```python
from build123d import *

# Parameters (mm, degrees)
SKETCH1_W               = 177.8
SKETCH1_H               = 317.5
BASE_DEPTH              = 6.35
HOLES_DEPTH             = 183.057944073
HOLES_DEPTH_BACK        = 183.057944073
SKETCH3_R               = 3.302
INNER_CUTOUT_DEPTH      = 183.057944073
INNER_CUTOUT_DEPTH_BACK = 183.057944073
FILLET1_R               = 6.35


with BuildPart() as part:
    # Sketch1 → Base (new body)
    with BuildSketch(Plane(origin=(0, 0, 0), x_dir=(1, 0, 0), z_dir=(0, 1, 0))):
        Rectangle(SKETCH1_W, SKETCH1_H)
    extrude(amount=BASE_DEPTH)

    # Sketch3 → Holes (cut, two sides: drawn at the far end of the back side and taken through both)
    with BuildSketch(Plane.XZ.offset(-HOLES_DEPTH_BACK)):
        with Locations(Location((-76.2, -146.05, 0), (0, 0, 270))):
            Circle(SKETCH3_R)
        with Locations(Location((76.2, -146.05, 0), (0, 0, 270))):
            Circle(SKETCH3_R)
        with Locations(Location((76.2, 133.35, 0), (0, 0, 270))):
            Circle(SKETCH3_R)
        with Locations(Location((-76.2, 133.35, 0), (0, 0, 270))):
            Circle(SKETCH3_R)
    extrude(amount=HOLES_DEPTH + HOLES_DEPTH_BACK, mode=Mode.SUBTRACT)

    # Sketch6 → Inner Cutout (cut, two sides: drawn at the far end of the back side and taken through both)
    with BuildSketch(Plane.XZ.offset(-INNER_CUTOUT_DEPTH_BACK)):
        with BuildLine():
            Line((-76.2, 120.65), (-76.2, -133.35))
            ThreePointArc((-76.2, -133.35), (-67.219743879, -137.069743879), (-63.5, -146.05))
            Line((-63.5, -146.05), (63.5, -146.05))
            ThreePointArc((63.5, -146.05), (67.219743879, -137.069743879), (76.2, -133.35))
            Line((76.2, -133.35), (76.2, 120.65))
            ThreePointArc((76.2, 120.65), (67.219743879, 124.369743879), (63.5, 133.35))
            Line((63.5, 133.35), (-63.5, 133.35))
            ThreePointArc((-63.5, 133.35), (-67.219743879, 124.369743879), (-76.2, 120.65))
        make_face()
    extrude(amount=INNER_CUTOUT_DEPTH + INNER_CUTOUT_DEPTH_BACK, mode=Mode.SUBTRACT)

    # Fillet1
    fillet1_edges = [part.edges().sort_by_distance(p)[0] for p in [
        (-76.2, 3.175, 120.65),
        (-63.5, 3.175, 133.35),
        (63.5, 3.175, 133.35),
        (76.2, 3.175, 120.65),
        (76.2, 3.175, -133.35),
        (63.5, 3.175, -146.05),
        (-63.5, 3.175, -146.05),
        (-76.2, 3.175, -133.35),
        (88.9, 3.175, 158.75),
        (-88.9, 3.175, 158.75),
        (-88.9, 3.175, -158.75),
        (88.9, 3.175, -158.75),
    ]]
    fillet(fillet1_edges, radius=FILLET1_R)


solid = part.part
```
Can you work these out from the model? Positions are in its coordinate system, mm. A direction names the side the tool comes from. Round coordinates to 2 decimals unless told otherwise and drop trailing zeros. Order: outer loops, then holes, each group sorted by start corner. A loop starts at its lowest first (then second) coordinate and runs counter-clockwise, first axis right, second up. Notation, with made-up numbers: (-9, 45) -> (42, 45) arc R24 cw to (42, 78) -> close; hole circle Ø2 at (25, 43). An arc over 180 degrees is marked (long way). Return JSON: item names as keys, results as strings. Group by question number.
1. If we section it at B-B, the plane y = 3: Write out the boundary of the cut face in (x, z).
2. I need wall thicknesses on line 1 (Z direction, x = -6, y = 4); line 2 (X direction, y = 3.25, z = -102.5); line 3 (X direction, y = 2, z = 132). Which ranges of each line are inside material? Lowest first, please. Write a range as [from, to].
3. If we section it at C-C, the plane z = -74.5: Write out the boundary of the cut face in (x, y).
4. If we section it at A-A, the plane x = 42.5: Write out the boundary of the cut face in (y, z).
5. We'd pull the mould along X, two halves only. Please class faces 1 (the face through (-61.861, 3.131, -144.916)), 2 (the face through (86.99, 3.22, 156.94)), 3 (the face through (-79, 6.35, 11)): released by +X, released by -X, zero draft, split by the parting line, or undercut.
6. Which directions (+Z, -Z, +X, -X, +Y, -Y) give clear straight access to the entire face, cutting with the end or side of a thin tool? Please do faces 4 (the face through (-75.003, 3.131, 119.1)), 5 (the face through (-1, 3, 158.75)).
Output values:
{
 "1": {"outline": "(-88.9, -152.4) arc R6.35 ccw to (-82.55, -158.75) -> (82.55, -158.75) arc R6.35 ccw to (88.9, -152.4) -> (88.9, 152.4) arc R6.35 ccw to (82.55, 158.75) -> (-82.55, 158.75) arc R6.35 ccw to (-88.9, 152.4) -> close; hole circle Ø6.6 at (-76.2, -146.05); hole circle Ø6.6 at (-76.2, 133.35); hole (-76.2, -128.09) arc R6.35 ccw to (-71.97, -134.08) arc R12.7 cw to (-64.23, -141.82) arc R6.35 ccw to (-58.24, -146.05) -> (58.24, -146.05) arc R6.35 ccw to (64.23, -141.82) arc R12.7 cw to (71.97, -134.08) arc R6.35 ccw to (76.2, -128.09) -> (76.2, 115.39) arc R6.35 ccw to (71.97, 121.38) arc R12.7 cw to (64.23, 129.12) arc R6.35 ccw to (58.24, 133.35) -> (-58.24, 133.35) arc R6.35 ccw to (-64.23, 129.12) arc R12.7 cw to (-71.97, 121.38) arc R6.35 ccw to (-76.2, 115.39) -> close; hole circle Ø6.6 at (76.2, -146.05); hole circle Ø6.6 at (76.2, 133.35)"},
 "2": {"line 1": "[-158.75, -146.05], [133.35, 158.75]", "line 2": "[-88.9, -76.2], [76.2, 88.9]", "line 3": "[-88.9, -79.21], [-73.19, -62.15], [62.15, 73.19], [79.21, 88.9]"},
 "3": {"outline": "(-88.9, 0) -> (-76.2, 0) -> (-76.2, 6.35) -> (-88.9, 6.35) -> close; (76.2, 0) -> (88.9, 0) -> (88.9, 6.35) -> (76.2, 6.35) -> close"},
 "4": {"outline": "(0, -158.75) -> (6.35, -158.75) -> (6.35, -146.05) -> (0, -146.05) -> close; (0, 133.35) -> (6.35, 133.35) -> (6.35, 158.75) -> (0, 158.75) -> close"},
 "5": {"face 1": "undercut", "face 2": "released by +X", "face 3": "zero draft"},
 "6": {"face 4": "+Y, -Y", "face 5": "+Z, +X, -X, +Y, -Y"}
}
